The figure shows three views and two pictorial views of one solid part (mm, origin at its lowest corner). Answer the questions. A direction names the side the tool comes from. Give positions to 0.01 mm unless a question says otherwise; leave off trailing zeros. Loops run counter-clockwise (first coordinate to the right, second up) from the corner with the lowest first, then second, coordinate; pieces in that order, holes last. Notation, with made-up numbers: M 73,-15 L 88,-15 A18 ccw 88,9 Z; hole C 41.5,51 d6. An arc over 180 degrees is marked long. Write item = value, one per line. Start each with the question number.
1. Section C-C on x = 17.5 is taken. Determine the outline of the cut face in (y, z).
2. Section A-A on y = 16.5 is taken. Determine the outline of the cut face in (x, z), plus the area to 3 significant figures.
3. Consider L1, parallel to X at y = 14, z = 4.75; L2, parallel to Y at x = 12.5, z = 7.5; L3, parallel to Y at x = 3, z = 22.75. Determine where each line is inside the solid, lowest interval first. Write a range as [from, to].
4. For the marked faces 1 and 2, determine the directions among +Z, -Z, +X, -X, +Y, -Y from which every point of the face is accessible in a straight line to the end or side of a thin tool.
5. The mould has two halves that part along X. Classify the marked faces 3, 4 and 5: released by +X, released by -X, zero draft, split by the parting line, or undercut.
6. Section D-D on y = 26 is taken. Determine the outline of the cut face in (x, z), plus the area to 3 significant figures.
7. Section B-B on z = 7.25 is taken. Determine the outline of the cut face in (x, y), plus the area to 3 significant figures.
8. Flat-ended cylindrical pins translate along their axes: pin 1 Ø8 at (x, y) = (15, 13) entering from +Z; pin 2 Ø5 at (x, z) = (32.5, 16) entering from +Y. Find the tip coordinate at first contact, or state that the pin passes through.
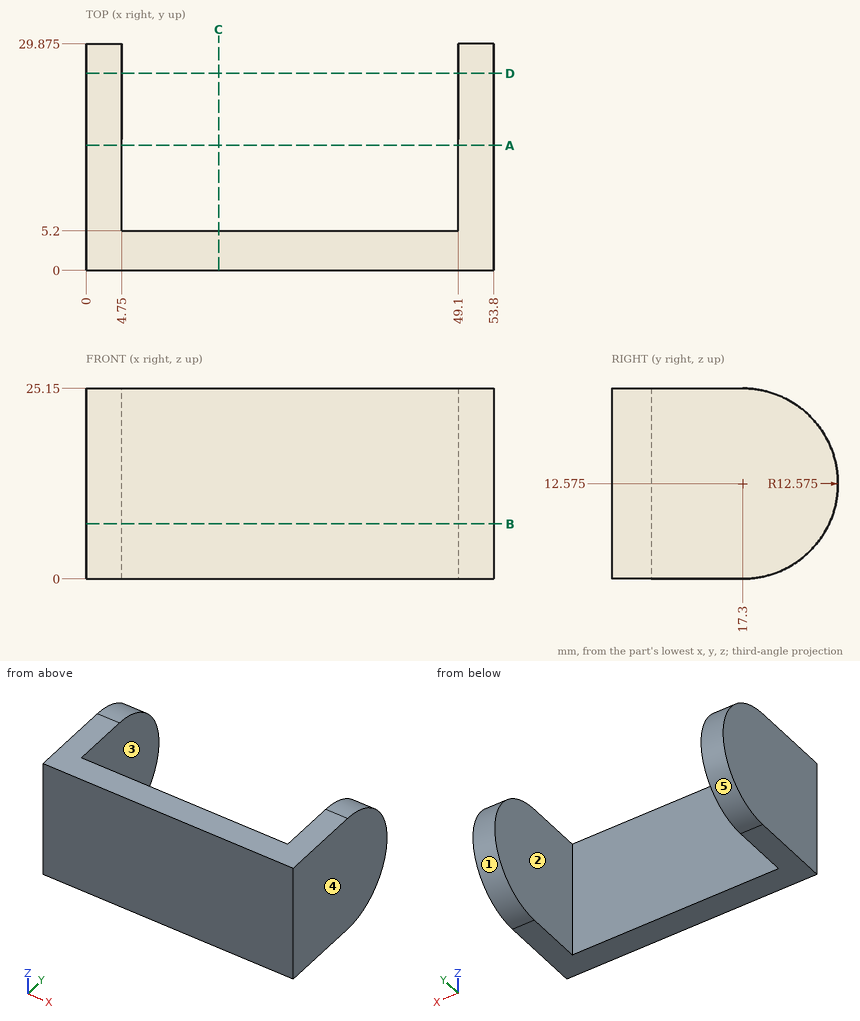
Verdict:
q1.outline = M 0,0 L 5.2,0 L 5.2,25.15 L 0,25.15 Z
q2.outline = M 0,0 L 4.75,0 L 4.75,25.15 L 0,25.15 Z; M 49.1,0 L 53.8,0 L 53.8,25.15 L 49.1,25.15 Z
q2.area = 238 mm2
q3.L1 = [0, 4.75], [49.1, 53.8]
q3.L2 = [0, 5.2]
q3.L3 = [0, 24.69]
q4.face_1 = +X, -X, +Y
q4.face_2 = +Z, -Z, +Y
q5.face_3 = undercut
q5.face_4 = released by +X
q5.face_5 = zero draft
q6.outline = M 0,3.5 L 4.75,3.5 L 4.75,21.65 L 0,21.65 Z; M 49.1,3.5 L 53.8,3.5 L 53.8,21.65 L 49.1,21.65 Z
q6.area = 172 mm2
q7.outline = M 0,0 L 53.8,0 L 53.8,28.69 L 49.1,28.69 L 49.1,5.2 L 4.75,5.2 L 4.75,28.69 L 0,28.69 Z
q7.area = 502 mm2
q8.pin_1 = through
q8.pin_2 = 5.2
